from build123d import *

# Parameters (mm, degrees)
BOSS_EXTRU_1_DEPTH = 10


with BuildPart() as part:
    # Esquisse1 → Boss.-Extru.1 (new body)
    with BuildSketch(Plane.XY):
        Polygon((-600, 0), (0, 0), (0, -125), (-215, -125), (-600, -31.25), align=None)
    extrude(amount=-BOSS_EXTRU_1_DEPTH)


solid = part.part
Check sheet for the modelled part. Datum: model origin and axes. Units: mm. Give positions to 0.01 mm unless a question says otherwise; leave off trailing zeros. Loops run counter-clockwise (first coordinate to the right, second up) from the corner with the lowest first, then second, coordinate; pieces in that order, holes last. Notation, with made-up numbers: M -31.75,44.25 L -8.75,44.25 A6 cw -8.75,48.25 Z; hole C -39,-25.5 d5. An arc over 180 degrees is marked long. Use a Markdown table: item, result. Add a question column.
Q1. Sectioned sample at C-C, the plane x = -465. Record the cut outline in (y, z), then the cut area to 3 significant figures.
Q2. Sectioned sample at A-A, the plane z = -4. Record the cut outline in (x, y), then the cut area to 3 significant figures.
Q3. Sectioned sample at B-B, the plane y = -110. Record the cut outline in (x, z), then the cut area to 3 significant figures.
Q4. Scan lines: line 1 along Y through (x, z) = (-378.5, -1.75); line 2 along Y through (x, z) = (-403, -0.25). Record each from-to range of solid material in increasing order. Write a range as [from, to].
Verdict:
| question | item | result |
|---|---|---|
| 1 | outline | M -64.12,-10 L 0,-10 L 0,0 L -64.12,0 Z |
| 1 | area | 641 mm^2 |
| 2 | outline | M -600,-31.25 L -215,-125 L 0,-125 L 0,0 L -600,0 Z |
| 2 | area | 57,000 mm^2 |
| 3 | outline | M -276.6,-10 L 0,-10 L 0,0 L -276.6,0 Z |
| 3 | area | 2,770 mm^2 |
| 4 | line 1 | [-85.19, 0] |
| 4 | line 2 | [-79.22, 0] |
